Could you check a few things on this model? Use its own coordinates, in mm. A direction names the side the tool comes from. Round coordinates to 2 decimals unless told otherwise and drop trailing zeros. Loops run counter-clockwise (first coordinate to the right, second up) from the corner with the lowest first, then second, coordinate; pieces in that order, holes last. Notation, with made-up numbers: M 41.25,58.25 L 56.25,58.25 A26 cw 56.25,77.25 Z; hole C 5,55.5 d4. An arc over 180 degrees is marked long. Return JSON: item names as keys, results as strings. Group by question number.
Autodesk Inventor part; units mm, degrees
ref_plane "YZ Plane" through (0, 0, 0) normal (1, 0, 0) x (0, 1, 0)
ref_plane "XZ Plane" through (0, 0, 0) normal (0, 1, 0) x (-1, 0, 0)
ref_plane "XY Plane" through (0, 0, 0) normal (0, 0, 1) x (1, 0, 0)
sketch "Sketch1" plane through (0, 0, 0) normal (0, 1, 0) x (-1, 0, 0)
  line L0 (-12.2941, 0) -> (-17, 0)
  line L1 (-17, 0) -> (-17, 7.5)
  line L2 (0, 0) -> (-12.2941, 0)
  line L3 (-12.2941, 9) -> (-10.7238, 9)
  line L4 (-12.2941, 9) -> (-13.7941, 7.5)
  line L5 (-12.2941, 9) -> (-9.8817, 9) construction
  arc A0 (-10.7238, -9) -> (-10.7238, 9) centre (0, 0) ccw
  line L6 (-17, 7.5) -> (-13.7941, 7.5)
  line L7 (-17, 0) -> (-17, -7.5)
  line L8 (-12.2941, -9) -> (-10.7238, -9)
  line L9 (-12.2941, -9) -> (-13.7941, -7.5)
  line L10 (-12.2941, -9) -> (-9.8817, -9) construction
  line L11 (-17, -7.5) -> (-13.7941, -7.5)
  dimension "d3" = 9
  dimension "d4" = 135
extrude "Extrusion1" add sketch "Sketch1" along normal blind 19
sketch "Sketch2" plane through (0, 19, 0) normal (0, 1, 0) x (1, 0, 0)
  circle A0 centre (-7.5, 0) radius 4.6
  circle A1 centre (-7.5, 0) radius 2.5
  arc A2 (10.7238, 9) -> (10.7238, -9) centre (0, 0) ccw
  line L0 (-6, -2) -> (-6, 2)
  line L1 (-9, 2) -> (-9, -2)
  circle A3 centre (0, -17.5) radius 2
  arc A4 (-3.5, -17.5) -> (3.5, -17.5) centre (0, -17.5) ccw
  line L2 (-3.5, -17.5) -> (-3.5, -13.5554)
  line L3 (3.5, -17.5) -> (3.5, -13.5554)
  arc A5 (-3.5, -13.5554) -> (3.5, -13.5554) centre (0, 0) ccw
  line L4 (0, 0) -> (2, 0)
  arc A6 (10.7238, 9) -> (10.7238, -9) centre (0, 0) ccw
  circle A7 centre (0, 17.5) radius 2
  arc A8 (3.5, 17.5) -> (-3.5, 17.5) centre (0, 17.5) ccw
  line L5 (-3.5, 17.5) -> (-3.5, 13.5554)
  line L6 (3.5, 17.5) -> (3.5, 13.5554)
  arc A9 (3.5, 13.5554) -> (-3.5, 13.5554) centre (0, 0) ccw
  point P0 (-7.5, -3.3735)
  dimension "d7" = 5
  dimension "d8" = 9.2
  dimension "d9" = 0
  dimension "d10" = 7.5
  dimension "d12" = 0
  dimension "d13" = 3
  dimension "d14" = 4
  dimension "d15" = 0
  dimension "d16" = 17.5
  dimension "d17" = 7
extrude "Extrusion2" add sketch "Sketch2" against normal blind 1 contours A2 L3 A4 L2 | A2 L5 A8 L6
extrude "Extrusion3" add sketch "Sketch2" along normal blind 9 contours L0 A1 L1
extrude "Extrusion4" add sketch "Sketch2" along normal blind 3 contours A1 L0 | L0 A1 L1 | L1 A1
extrude "Extrusion5" add sketch "Sketch2" along normal blind 1.5 contours A0
sketch "Sketch4" plane through (0, 19, 0) normal (0, 1, 0) x (1, 0, 0)
  point P0 (0, 0)
properties part number "stepper_motor"
1. If we section it at C-C, the plane z = 0: Please give me the cut outline in (x, y).
2. If we section it at D-D, the plane x = -11.5: Please give me the cut outline in (y, z).
3. I'm going to push flat-ended pins straight in: pin 1 Ø1.1 at (y, z) = (18.5, -15) entering from -X; pin 2 Ø2 at (x, z) = (6, -11.5) entering from +Y; pin 3 Ø1.2 at (y, z) = (25.5, -0.5) entering from -X; pin 4 Ø2.5 at (x, z) = (0, -17.5) entering from +Y. Where does each tip first touch, or does it pass through?
4. We'd pull the mould along Z, two halves only. Please class faces 1 (the face through (-0.26, 18.507, -19.483)), 2 (the face through (12, 9, 9)), 3 (the face through (-3.25, 19.74, -1.76)): +Z half, -Z half, draft (parallel to the pull), parting line (faces both ways), or undercut.
5. On a 3-axis mill with a long thin cutter (end or side, diameter ignored), from which of +Z, -Z, +X, -X, +Y, -Y can I reach the whole of each face in a straight line? I mean faces 4 (the face through (-14, 9, 0)), 5 (the face through (-9.4, 22, 0)), 6 (the face through (-6.16, 23.36, 2.11)), 7 (the face through (3.5, 18.5, 15.6)). Say none if no direction works.
6. I need wall thicknesses on probe 1 along X at (y, z) = (18.6, -17.5); probe 2 along Y at (x, z) = (-5, -8.5); probe 3 along Y at (x, z) = (-11, 1). Which ranges of each line are inside material? Lowest first, please.
7. If we section it at B-B, the plane y = 17.25: Please give me the cut outline in (x, z), then the cut area to 3 significant figures.
8. If we section it at A-A, the plane x = 0: Please give me the cut outline in (y, z), then the cut area to 3 significant figures.
Geometry results:
{
 "1": {"outline": "M -14,0 L 17,0 L 17,19 L -2.9,19 L -2.9,20.5 L -5,20.5 L -5,22 L -6,22 L -6,28 L -9,28 L -9,22 L -10,22 L -10,20.5 L -12.1,20.5 L -12.1,19 L -14,19 Z"},
 "2": {"outline": "M 0,-7.98 L 19,-7.98 L 19,-2.27 L 20.5,-2.27 L 20.5,2.27 L 19,2.27 L 19,7.98 L 0,7.98 Z"},
 "3": {"pin 1": "x = -3.5", "pin 2": "y = 19", "pin 3": "x = -9", "pin 4": "through"},
 "4": {"face 1": "undercut", "face 2": "+Z half", "face 3": "parting line"},
 "5": {"face 4": "-Y", "face 5": "+Z, -Z, -X, +Y", "face 6": "+Y", "face 7": "+Z, +X, +Y, -Y"},
 "6": {"probe 1": "-3.5 to -2, 2 to 3.5", "probe 2": "0 to 19", "probe 3": "0 to 20.5"},
 "7": {"outline": "M 10.72,-9 L 12.29,-9 L 13.79,-7.5 L 17,-7.5 L 17,7.5 L 13.79,7.5 L 12.29,9 L 10.72,9 A14 ccw long Z", "area": "677 mm^2"},
 "8": {"outline": "M 0,-14 L 18,-14 L 18,-15.5 L 19,-15.5 L 19,15.5 L 18,15.5 L 18,14 L 0,14 Z; M 18,-21 L 19,-21 L 19,-19.5 L 18,-19.5 Z; M 18,19.5 L 19,19.5 L 19,21 L 18,21 Z", "area": "538 mm^2"}
}
